Read the model definition and answer for the solid it produces. Units are mm, in the model's axes. A direction names the side the tool comes from. Round coordinates to 2 decimals unless told otherwise and drop trailing zeros. Loops run counter-clockwise (first coordinate to the right, second up) from the corner with the lowest first, then second, coordinate; pieces in that order, holes last. Notation, with made-up numbers: (19.5, 28.5) - (26.5, 28.5) arc R15 cw to (26.5, 40.5) - close; hole circle Ø1 at (27, 22.25). An arc over 180 degrees is marked (long way). Answer as CSV lines item,"result".
Autodesk Inventor part; units mm, degrees
ref_plane "YZ Plane" through (0, 0, 0) normal (1, 0, 0) x (0, 1, 0)
ref_plane "XZ Plane" through (0, 0, 0) normal (0, 1, 0) x (-1, 0, 0)
ref_plane "XY Plane" through (0, 0, 0) normal (0, 0, 1) x (1, 0, 0)
sketch "Sketch1" plane through (0, 0, 0) normal (0, 1, 0) x (-1, 0, 0)
  line L0 (-25, -37.5) -> (25, -37.5)
  line L1 (25, -37.5) -> (25, 30.5)
  line L2 (25, 30.5) -> (-25, 30.5)
  line L3 (-25, 30.5) -> (-25, -37.5)
  line L4 (-25, -37.5) -> (25, 30.5) construction
  line L5 (25, -37.5) -> (-25, 30.5) construction
  point P0 (0, -3.5)
  point P1 (0, -3.5)
  point P2 (0, -3.5)
  dimension "d2" = 1.6
  dimension "d0" = 68
  dimension "d1" = 50
extrude "Extrusion1" add sketch "Sketch1" along normal blind 1.6
sketch "Sketch2" plane through (0, 0, 0) normal (0, -1, 0) x (1, 0, 0)
  line L0 (25, 30.5) -> (25, -37.5)
  line L1 (25, -29.5) -> (34, -29.5)
  line L2 (34, -29.5) -> (34, 30.5)
  line L3 (34, 30.5) -> (25, 30.5)
  line L4 (25, 30.5) -> (25, -29.5)
  line L5 (-25, -37.5) -> (-25, 30.5)
  line L6 (-25, -29.5) -> (-34, -29.5)
  line L7 (-34, -29.5) -> (-34, 30.5)
  line L8 (-34, 30.5) -> (-25, 30.5)
  line L9 (-25, 30.5) -> (-25, -29.5)
  line L10 (25, -37.5) -> (-25, -37.5)
  line L11 (-7.5, 37.5) -> (7.5, 37.5)
  line L12 (7.5, 37.5) -> (7.5, 30.5)
  line L13 (7.5, 30.5) -> (-7.5, 30.5)
  line L14 (-7.5, 30.5) -> (-7.5, 37.5)
  line L15 (-7.5, 37.5) -> (7.5, 30.5) construction
  line L16 (7.5, 37.5) -> (-7.5, 30.5) construction
  line L17 (-25, 30.5) -> (25, 30.5)
  point P0 (0, 0)
  point P1 (25, 28.5)
  point P2 (25, -35.5)
  point P3 (-25, -35.5)
  point P4 (-25, 28.5)
  point P5 (-23, 30.5)
  point P6 (23, 30.5)
  point P7 (23, -37.5)
  point P8 (-23, -37.5)
  point P9 (25, 23.5)
  point P10 (-25, 23.5)
  point P11 (25, 28.5)
  point P12 (-25, 28.5)
  point P13 (0, 34)
  point P14 (0, 34)
  point P15 (0, 30.5)
  dimension "d5" = 9
  dimension "d6" = 9
  dimension "d8" = 8
  dimension "d12" = 15
  dimension "d13" = 7
extrude "Extrusion2" add sketch "Sketch2" against normal up to surface (1.6 mm away) contours L3 L2 L1 L0 | L13 L14 L11 L12 | L5 L6 L7 L8
fillet "Fillet2" radius 1 12 edges at (-34, 0.8, 30.5) (-25, 0.8, -29.5) (-34, 0.8, -29.5) (25, 0.8, -29.5) (34, 0.8, -29.5) (34, 0.8, 30.5) (25, 0.8, -37.5) (-25, 0.8, -37.5) (7.5, 0.8, 30.5) (7.5, 0.8, 37.5) (-7.5, 0.8, 37.5) (-7.5, 0.8, 30.5)
properties part number "MainBoard"
1) A tool of negligible diameter and unlimited length cuts with its end or side. For faces 1 (the face through (-25, 1, -34)), 2 (the face through (7.5, 1, 34)), 3 (the face through (25, 1, -33)), from which of +Z, -Z, +X, -X, +Y, -Y can it reach the whole face along a straight path? Write none if from no direction.
Entries:
face 1,"-Z, -X, +Y, -Y"
face 2,"+Z, +X, +Y, -Y"
face 3,"-Z, +X, +Y, -Y"
2) A cutting plane is placed at A-A, the plane y = 0.4. Determine the outline of the cut face in (x, z), plus the area to 3 significant figures.
Entries:
outline,"(-34, -28.5) arc R1 ccw to (-33, -29.5) - (-26, -29.5) arc R1 cw to (-25, -30.5) - (-25, -36.5) arc R1 ccw to (-24, -37.5) - (24, -37.5) arc R1 ccw to (25, -36.5) - (25, -30.5) arc R1 cw to (26, -29.5) - (33, -29.5) arc R1 ccw to (34, -28.5) - (34, 29.5) arc R1 ccw to (33, 30.5) - (8.5, 30.5) arc R1 cw to (7.5, 31.5) - (7.5, 36.5) arc R1 ccw to (6.5, 37.5) - (-6.5, 37.5) arc R1 ccw to (-7.5, 36.5) - (-7.5, 31.5) arc R1 cw to (-8.5, 30.5) - (-33, 30.5) arc R1 ccw to (-34, 29.5) - close"
area,"4,580 mm^2"
3) A cutting plane is placed at B-B, the plane x = 16.5. Determine the outline of the cut face in (y, z).
Entries:
outline,"(0, -37.5) - (1.6, -37.5) - (1.6, 30.5) - (0, 30.5) - close"
4) Find the intervals of material crossed by line 1 (Z direction, x = 31, y = 1.3); line 2 (X direction, y = 0.5, z = 33); line 3 (Z direction, x = -21, y = 0.8), in increasing order.
Entries:
line 1,"z = -29.5 to 30.5"
line 2,"x = -7.5 to 7.5"
line 3,"z = -37.5 to 30.5"
5) The mould has two halves that part along Y. Classify faces 4 (the face through (0, 0, 1)), 5 (the face through (-34, 1, 0)), 6 (the face through (0, 1.6, 1)): pulls with the +Y half, pulls with the -Y half, needs draft (parallel to the pull), parting line crosses it, or undercut.
Entries:
face 4,"pulls with the -Y half"
face 5,"needs draft"
face 6,"pulls with the +Y half"
6) Each of these flat-tipped pins is pushed along its axis until it touches: P1, Ø0.5, axis at y = 1, z = 34, coming from the -X side; P2, Ø0.5, axis at x = -21, y = 1, coming from the +Z side; P3, Ø0.5, axis at x = 29.5, y = 0.5, coming from the -Z side. Where does it stop, or does it pass through?
Entries:
P1,"stops at x = -7.5"
P2,"stops at z = 30.5"
P3,"stops at z = -29.5"
